Build history of the part. All positions in model axes, mm. Face numbers are marked on the shaded views. A direction names the side the tool comes from. Coordinates: 2 decimals unless noted, no trailing zeros. Write each loop counter-clockwise with the first axis right and the second up, starting at its lowest first coordinate (ties: lowest second). Pieces come first, ordered by that corner, then holes. Notation, with made-up numbers: M -21.5,-16 L -16.5,-16 A23 ccw -16.5,20 Z; hole C 47.25,45 d3. An arc over 180 degrees is marked long. Use CSV: the item, a comma, the result in double quotes. Start each with the question number.
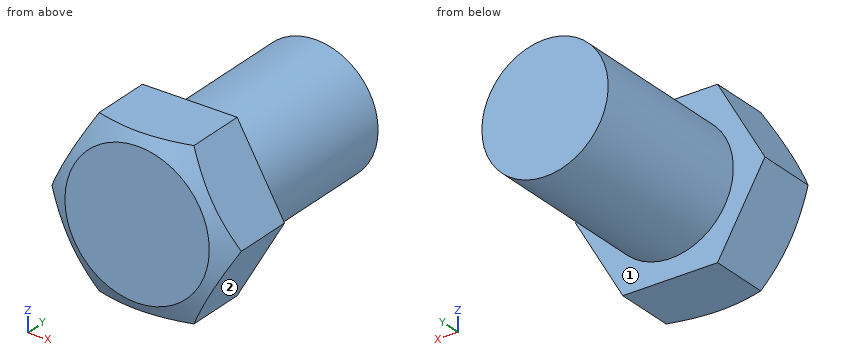
```python
from build123d import *

# Parameters (mm, degrees)
EXTRUDE_1_DEPTH     = 8
SKETCH_2_R          = 7
EXTRUDE_2_DEPTH     = 19
SKETCH_3_OUTSIDE_W  = 35.944
SKETCH_3_OUTSIDE_H  = 33.13
SKETCH_3_OUTSIDE_R  = 8
CUT_EXTRUDE_2_DEPTH = 1.5
CUT_EXTRUDE_2_TAPER = 60


with BuildPart() as part:
    # Эскиз1 → Бобышка-Вытянуть1 (new body)
    with BuildSketch(Plane(origin=(0, 0, 0), x_dir=(1, 0, 0), z_dir=(0, 1, 0))):
        Polygon((10.5, 0), (5.25, 9.09326674), (-5.25, 9.09326674), (-10.5, 0), (-5.25, -9.09326674), (5.25, -9.09326674), align=None)
    extrude(amount=EXTRUDE_1_DEPTH)

    # Эскиз2 → Бобышка-Вытянуть2 (add)
    with BuildSketch(Plane(origin=(0, 8, 0), x_dir=(1, 0, 0), z_dir=(0, 1, 0))):
        Circle(SKETCH_2_R)
    extrude(amount=EXTRUDE_2_DEPTH)

    # Эскиз3 outside → Вырез-Вытянуть2 (cut)
    with BuildSketch(Plane.XZ):
        Rectangle(SKETCH_3_OUTSIDE_W, SKETCH_3_OUTSIDE_H)
        Circle(SKETCH_3_OUTSIDE_R, mode=Mode.SUBTRACT)
    extrude(amount=-CUT_EXTRUDE_2_DEPTH, taper=CUT_EXTRUDE_2_TAPER, mode=Mode.SUBTRACT)


solid = part.part
```
1. Slice it at A-A (x = 0). List the corners of the cut face in (y, z).
2. Slice it at B-B (y = 9.75). List the corners of the cut face in (x, z), and give its area (3 significant figures).
3. Flat gauge pins, fed straight in: pin 1 (6 mm diameter, centred on y = 20, z = -2.5, fed in from -X); pin 2 (1.5 mm diameter, centred on y = 14, z = 6.5, fed in from +X); pin 3 (8 mm diameter, centred on x = -1.5, y = 23.5, fed in from +Z). Where does each tip first touch, or does it go through?
4. 3-axis set-ups, long thin cutter, end or side, ignore diameter. For the marked faces 1 and 2: which of +Z, -Z, +X, -X, +Y, -Y reach the whole face in a straight line?
5. Drill centre lines: line 1 along X through (y, z) = (24.5, 0.25); line 2 along Y through (x, z) = (-2.5, 7.25); line 3 along X through (y, z) = (24.75, -3.25). Where is each one in solid material? Low to high. Write a range as from..to.
Established:
1,outline,"M 0,-8 L 0.63,-9.09 L 8,-9.09 L 8,-7 L 27,-7 L 27,7 L 8,7 L 8,9.09 L 0.63,9.09 L 0,8 Z"
2,outline,"C 0,0 d14"
2,area,"154 mm2"
3,pin 1,"stops at x = -7"
3,pin 2,"stops at x = 3.99"
3,pin 3,"stops at z = 7"
4,face 1,"+Y"
4,face 2,"-Z, +X, +Y, -Y"
5,line 1,"x = -7..7"
5,line 2,"y = 0..8"
5,line 3,"x = -6.2..6.2"
